from build123d import *

# Parameters (mm, degrees)
ESQUISSE1_R        = 0.75
BOSS_EXTRU_1_DEPTH = 3.3
BOSS_EXTRU_2_DEPTH = 3.3


with BuildPart() as part:
    # Balayage1: sweep along a curve in space
    with BuildLine() as balayage1_path:
        Line((0, 0, 0), (20.71, 0, 0))
        Line((20.71, 0, 0), (20.71, 56.56, 0))
        Line((20.71, 56.56, 0), (20.71, 56.56, 19.48))
        Line((20.71, 56.56, 19.48), (3.95, 56.56, 19.48))
        Line((3.95, 56.56, 19.48), (3.95, 50.06, 19.48))
    # Esquisse1 → Balayage1 (sweep)
    with BuildSketch(Plane(origin=(0, 0, 0), x_dir=(0, 0, -1), z_dir=(1, 0, 0))):
        Circle(ESQUISSE1_R)
    sweep(path=balayage1_path.line, transition=Transition.RIGHT)

    # Esquisse2 → Boss.-Extru.1 (add)
    with BuildSketch(Plane.ZY):
        with BuildLine():
            Line((-0.693559654, 3.410973121), (-0.033559654, 3.410973121))
            Line((-0.033559654, 3.410973121), (0.052886955, 3.410800656))
            ThreePointArc((0.052886955, 3.410800656), (0.152585895, 3.390814178), (0.237103646, 3.334280227))
            Line((0.237103646, 3.334280227), (0.840288261, 2.731095613))
            ThreePointArc((0.840288261, 2.731095613), (0.915698502, 2.601090787), (0.916612811, 2.450800656))
            Line((0.916612811, 2.450800656), (0.907780092, -2.544199344))
            ThreePointArc((0.907780092, -2.544199344), (0.890549579, -2.690753591), (0.840288109, -2.829493716))
            Line((0.840288109, -2.829493716), (0.229663651, -3.425976039))
            ThreePointArc((0.229663651, -3.425976039), (0.148335129, -3.479631619), (0.052886955, -3.499199344))
            Line((0.052886955, -3.499199344), (-0.683559654, -3.499199344))
            ThreePointArc((-0.683559654, -3.499199344), (-0.867407417, -3.423047107), (-0.943559654, -3.239199344))
            Line((-0.943559654, -3.239199344), (-0.943559654, 3.142794831))
            ThreePointArc((-0.943559654, 3.142794831), (-0.871366367, 3.326111221), (-0.693559654, 3.410973121))
        make_face()
    extrude(amount=BOSS_EXTRU_1_DEPTH)

    # Esquisse8 → Boss.-Extru.2 (add)
    with BuildSketch(Plane.XZ.offset(-50.06)):
        with BuildLine():
            Line((0.626082703, 19.600404574), (0.626082703, 18.6131001))
            ThreePointArc((0.626082703, 18.6131001), (0.629011635, 18.606029032), (0.636082703, 18.6031001))
            Line((0.636082703, 18.6031001), (7.516082703, 18.6031001))
            ThreePointArc((7.516082703, 18.6031001), (7.523153771, 18.606029032), (7.526082703, 18.6131001))
            Line((7.526082703, 18.6131001), (7.526082703, 19.600404544))
            ThreePointArc((7.526082703, 19.600404544), (7.524677417, 19.603797205), (7.521284755, 19.605202492))
            Line((7.521284755, 19.605202492), (6.680559004, 20.450070379))
            ThreePointArc((6.680559004, 20.450070379), (6.677327923, 20.452237942), (6.673512365, 20.452999341))
            Line((6.673512365, 20.452999341), (1.47867747, 20.452999341))
            Line((1.47867747, 20.452999341), (0.633809583, 19.612273589))
            ThreePointArc((0.633809583, 19.612273589), (0.629318413, 19.606747742), (0.626082703, 19.600404574))
        make_face()
    extrude(amount=BOSS_EXTRU_2_DEPTH)


solid = part.part
Check sheet for the modelled part. Datum: model origin and axes. Units: mm. A direction names the side the tool comes from. Coordinates: 2 decimals unless noted, no trailing zeros. Loops run counter-clockwise (first coordinate to the right, second up) from the corner with the lowest first, then second, coordinate; pieces in that order, holes last. Notation, with made-up numbers: (24, -21) -> (50, -21) arc R21 ccw to (50, -16) -> close; hole circle Ø4 at (51.25, 56). An arc over 180 degrees is marked (long way). Write item = value, one per line. Start each with the question number.
1. Section check C-C on x = 20.71. Record the cut outline in (y, z).
2. Section check D-D on z = 16. Record the cut outline in (x, y), then the cut area to 3 significant figures.
3. Section check B-B on y = 56.56. Record the cut outline in (x, z).
4. Material ranges on line 1 (Y direction, x = 18.25, z = 0), recorded low to high.
5. Tool access check on faces 1 (the cylindrical face through (12.2, 57.25, 19.77)), 2 (the flat face through (4, 46.76, 20)). Record the directions out of +Z, -Z, +X, -X, +Y, -Y that give a thin tool (end or side, any length) a straight path to the whole face; none if there is none.
6. Section check A-A on x = 3.95. Record the cut outline in (y, z), then the cut area to 3 significant figures.
7. Depth check by flat-ended pin: P1, Ø1.1, axis at y = 49, z = 19, coming from the -X side; P2, Ø0.6, axis at x = 3, z = 19, coming from the -Y side; P3, Ø2.5, axis at x = 5.5, y = 48, coming from the -Z side. Enter the tip coordinate at first touch or a pass-through.
Responses:
q1.outline = (0, -0.75) -> (57.31, -0.75) -> (57.31, 19.48) arc R0.75 ccw to (55.81, 19.48) -> (55.81, 0.75) -> (0, 0.75) arc R0.75 ccw to start
q2.outline = circle Ø1.5 at (20.71, 56.56)
q2.area = 1.77 mm2
q3.outline = (3.95, 18.73) -> (19.96, 18.73) -> (19.96, 0) arc R0.75 ccw to (21.46, 0) -> (21.46, 20.23) -> (3.95, 20.23) arc R0.75 ccw to start
q4.line_1 = -0.75 to 0.75
q5.face_1 = none
q5.face_2 = +Z, -Z, +X, -X, -Y
q6.outline = circle Ø1.5 at (0, 0); (46.76, 18.6) -> (50.06, 18.6) -> (50.06, 18.73) -> (56.56, 18.73) arc R0.75 ccw to (56.56, 20.23) -> (50.06, 20.23) -> (50.06, 20.45) -> (46.76, 20.45) -> close
q6.area = 18.5 mm2
q7.P1 = 0.63
q7.P2 = 46.76
q7.P3 = 18.6
